Here's how the part is built. I have some questions about the finished solid (model axes, mm). Face numbers are marked on the shaded views. A direction names the side the tool comes from. Round coordinates to 2 decimals unless told otherwise and drop trailing zeros. Write each loop counter-clockwise with the first axis right and the second up, starting at its lowest first coordinate (ties: lowest second). Pieces come first, ordered by that corner, then holes. Notation, with made-up numbers: (82.25, 14) -> (119.25, 14) arc R12 ccw to (119.25, 30) -> close; hole circle Ø2 at (86.5, 58.5). An arc over 180 degrees is marked (long way). Answer as CSV lines item,"result".
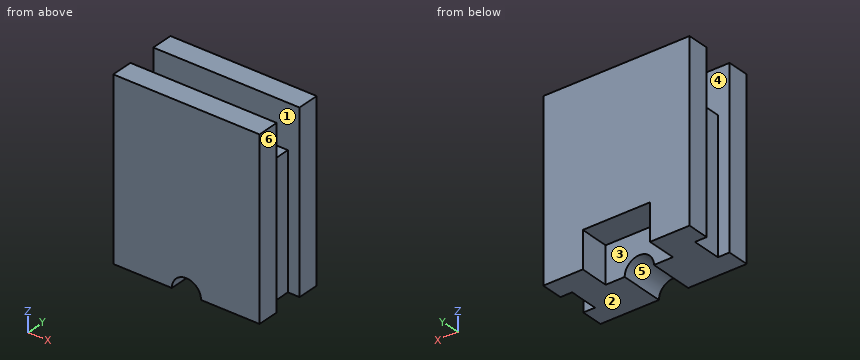
from build123d import *

# Parameters (mm, degrees)
EXTRUDE_1_DEPTH     = 60
SKETCH_2_W          = 15
SKETCH_2_H          = 10
CUT_EXTRUDE_1_DEPTH = 77.630607462
SKETCH_4_R          = 5
CUT_EXTRUDE_2_DEPTH = 70.641941386
SKETCH_5_W          = 23
SKETCH_5_H          = 25
CUT_EXTRUDE_3_DEPTH = 10


with BuildPart() as part:
    # Эскиз1 → Бобышка-Вытянуть1 (new body)
    with BuildSketch(Plane.XY):
        Polygon((-25, -5), (-25, -12.5), (25, -12.5), (25, -5), (21, -5), (21, 5), (25, 5), (25, 12.5), (-25, 12.5), (-25, 5), (-21, 5), (-21, -5), align=None)
    extrude(amount=EXTRUDE_1_DEPTH)

    # Эскиз2 → Вырез-Вытянуть1 (cut, through all)
    with BuildSketch(Plane.ZY.offset(21)):
        with Locations((52.5, 0)):
            Rectangle(SKETCH_2_W, SKETCH_2_H)
    extrude(amount=-CUT_EXTRUDE_1_DEPTH, mode=Mode.SUBTRACT)

    # Эскиз4 → Вырез-Вытянуть2 (cut, through all)
    with BuildSketch(Plane(origin=(0, 12.5, 0), x_dir=(1, 0, 0), z_dir=(0, 1, 0))):
        Circle(SKETCH_4_R)
    extrude(amount=-CUT_EXTRUDE_2_DEPTH, mode=Mode.SUBTRACT)

    # Эскиз5 → Вырез-Вытянуть3 (cut)
    with BuildSketch(Plane(origin=(0, 12.5, 0), x_dir=(1, 0, 0), z_dir=(0, 1, 0))):
        Rectangle(SKETCH_5_W, SKETCH_5_H)
    extrude(amount=-CUT_EXTRUDE_3_DEPTH, mode=Mode.SUBTRACT)


solid = part.part
Item 1: Suppose I cut it at C-C, the plane x = 9. List the corners of the cut face in (y, z) for me, then the cut area to 4 significant figures.
Results found:
outline,"(-12.5, 0) -> (2.5, 0) -> (2.5, 12.5) -> (12.5, 12.5) -> (12.5, 60) -> (5, 60) -> (5, 45) -> (-5, 45) -> (-5, 60) -> (-12.5, 60) -> close"
area,"1,225 mm²"
Item 2: For the marked faces 1, 2 and 3, which set-ups out of +Z, -Z, +X, -X, +Y, -Y let a thin tool reach every point of the face, with its end or its side?
Results found:
face 1,"+Z"
face 2,"-Z, +X, -X, +Y, -Y"
face 3,"-Z, +Y"
Item 3: Will these pins go through, and if not, where does the flat tip stop? pin 1 (5 mm diameter, centred on y = -0.5, z = 22, fed in from -X); pin 2 (8 mm diameter, centred on x = -4, y = 8.5, fed in from -Z); pin 3 (3 mm diameter, centred on x = 3, y = -2, fed in from +Z).
Results found:
pin 1,"stops at x = -21"
pin 2,"stops at z = 12.5"
pin 3,"stops at z = 45"
Item 4: I need wall thicknesses on L1, parallel to Y at x = 21, z = 46.5; L2, parallel to X at y = 5.25, z = 3.5; L3, parallel to Z at x = -20, y = -1.75. Which ranges of each line are inside material? Lowest first, please.
Results found:
L1,"y = -12.5 to -5, 5 to 12.5"
L2,"x = -25 to -11.5, 11.5 to 25"
L3,"z = 0 to 45"
Item 5: If we mould it in two halves opening along X, with no side actions, what happens to the marked faces 4, 5 and 6? For each: pulls with the +X half, pulls with the -X half, needs draft (parallel to the pull), parting line crosses it, or undercut.
Results found:
face 4,"needs draft"
face 5,"undercut"
face 6,"pulls with the +X half"
Item 6: Suppose I cut it at B-B, the plane y = 6. List the corners of the cut face in (x, z) for me.
Results found:
outline,"(-25, 0) -> (-11.5, 0) -> (-11.5, 12.5) -> (11.5, 12.5) -> (11.5, 0) -> (25, 0) -> (25, 60) -> (-25, 60) -> close"
Item 7: Suppose I cut it at D-D, the plane z = 32. List the corners of the cut face in (x, y) for me, then the cut area to 3 significant figures.
Results found:
outline,"(-25, -12.5) -> (25, -12.5) -> (25, -5) -> (21, -5) -> (21, 5) -> (25, 5) -> (25, 12.5) -> (-25, 12.5) -> (-25, 5) -> (-21, 5) -> (-21, -5) -> (-25, -5) -> close"
area,"1,170 mm²"
Item 8: Suppose I cut it at A-A, the plane z = 4. List the corners of the cut face in (x, y) for me.
Results found:
outline,"(-25, -12.5) -> (-3, -12.5) -> (-3, 2.5) -> (-11.5, 2.5) -> (-11.5, 12.5) -> (-25, 12.5) -> (-25, 5) -> (-21, 5) -> (-21, -5) -> (-25, -5) -> close; (3, -12.5) -> (25, -12.5) -> (25, -5) -> (21, -5) -> (21, 5) -> (25, 5) -> (25, 12.5) -> (11.5, 12.5) -> (11.5, 2.5) -> (3, 2.5) -> close"
